Autodesk Inventor part; units mm, degrees
ref_plane "YZ Plane" through (0, 0, 0) normal (1, 0, 0) x (0, 1, 0)
ref_plane "XZ Plane" through (0, 0, 0) normal (0, 1, 0) x (-1, 0, 0)
ref_plane "XY Plane" through (0, 0, 0) normal (0, 0, 1) x (1, 0, 0)
sketch "Sketch1" plane through (0, 0, 0) normal (0, 0, 1) x (1, 0, 0)
  circle A0 centre (0, 0) radius 4
  circle A1 centre (0, 0) radius 40 construction
  circle A2 centre (0, 0) radius 42 construction
  arc A3 (42, 0) -> (-42, 0) centre (0, 0) ccw
  line L0 (-42, 0) -> (-52, 0)
  line L1 (-52, 0) -> (-52, 50)
  line L2 (-52, 50) -> (52, 50)
  line L3 (52, 50) -> (52, 0)
  line L4 (52, 0) -> (42, 0)
  line L5 (-52, 0) -> (-42, 0)
  line L6 (-42, 0) -> (-42, -40)
  line L7 (-42, -40) -> (-52, -40)
  line L8 (-52, -40) -> (-52, 0)
  line L9 (52, 0) -> (42, 0)
  line L10 (42, 0) -> (42, -40)
  line L11 (42, -40) -> (52, -40)
  line L12 (52, -40) -> (52, 0)
  dimension "d0" = 8
  dimension "d1" = 80
  dimension "d2" = 2
  dimension "d3" = 50
  dimension "d4" = 10
  dimension "d5" = 40
extrude "Extrusion1" add sketch "Sketch1" along normal mid plane 7 contours A3 L0 L1 L2 L3 L4 | L4 L12 L11 L10 | L6 L7 L8 L0
sketch "Sketch2" plane through (0, 0, 3.5) normal (0, 0, 1) x (1, 0, 0)
  line L0 (42, 0) -> (42, -40)
  line L1 (42, -40) -> (52, -40)
  line L2 (52, -40) -> (52, 50)
  line L3 (52, 50) -> (-52, 50)
  line L4 (-52, 50) -> (-52, -40)
  line L5 (-52, -40) -> (-42, -40)
  line L6 (-42, -40) -> (-42, 0)
  arc A0 (42, 0) -> (-42, 0) centre (0, 0) ccw
  arc A1 (38, 0) -> (-38, 0) centre (0, 0) ccw
  line L7 (-38, 0) -> (-38, -40)
  line L8 (-38, -40) -> (-42, -40)
  line L9 (38, 0) -> (38, -40)
  line L10 (42, -40) -> (52, -40)
  line L11 (38, -40) -> (42, -40)
  dimension "d11" = 76
extrude "Extrusion2" add sketch "Sketch2" along normal blind 5
sketch "Sketch3" plane through (0, 0, 8.5) normal (0, 0, 1) x (1, 0, 0)
  line L0 (47, -25) -> (-47, -25) construction
  line L1 (-47, -25) -> (-47, 25) construction
  line L2 (-47, 25) -> (47, 25) construction
  line L3 (47, 25) -> (47, -25) construction
  line L4 (47, -25) -> (-47, 25) construction
  line L5 (-47, -25) -> (47, 25) construction
  arc A0 (42, 0) -> (-42, 0) centre (0, 0) ccw construction
  line L6 (-42, -40) -> (-42, 0) construction
  line L7 (42, 0) -> (42, -40) construction
  circle A1 centre (-47, 25) radius 2
  circle A2 centre (-47, -25) radius 2
  circle A3 centre (47, -25) radius 2
  circle A4 centre (47, 25) radius 2
  dimension "d12" = 4
  dimension "d13" = 5
  dimension "d14" = 50
extrude "Extrusion3" cut sketch "Sketch3" against normal through all
sketch "Sketch4" plane through (0, 0, 8.5) normal (0, 0, 1) x (1, 0, 0)
  circle A0 centre (-30, 42) radius 4
  circle A1 centre (30, 42) radius 4
  point P0 (0, 0)
extrude "Extrusion4" cut sketch "Sketch4" against normal through all
sketch "Sketch5" plane through (42, -40, -3.5) normal (0, -1, 0) x (1, 0, 0)
  line L0 (10, 0) -> (10, 12) construction
  line L1 (-4, 12) -> (10, 12) construction
  line L2 (-4, 7) -> (-4, 12)
  line L3 (-4, 7) -> (0, 7)
  line L4 (0, 0) -> (0, 7)
  line L5 (10, 0) -> (0, 0) construction
  line L6 (0, 0) -> (0, 7) construction
  line L7 (0, 3.5) -> (-3, 3.5) construction
  circle A0 centre (-3, 3.5) radius 3
  line L8 (-4, 12) -> (-8, 12)
  line L9 (-80, 12) -> (-4, 12)
  line L10 (-8, 12) -> (-8, 0)
  line L11 (-8, 0) -> (0, 0)
  point P0 (-42, 3.5)
  dimension "d19" = 6
  dimension "d20" = 4
extrude "Extrusion5" add sketch "Sketch5" against normal blind 10
mirror "Mirror1" about plane through (0, 0, 0) normal (1, 0, 0) of "Extrusion5"
fillet "Fillet1" radius 20 2 edges at (52, 50, 2.5) (-52, 50, 2.5)
fillet "Fillet2" radius 5 2 edges at (52, -40, 2.5) (-52, -40, 2.5)
properties part number "frame top"
CAD build for the part. Positions are in the model's coordinates, mm. A direction names the side the tool comes from. Round coordinates to 2 decimals unless told otherwise and drop trailing zeros. Write each loop counter-clockwise with the first axis right and the second up, starting at its lowest first coordinate (ties: lowest second). Pieces come first, ordered by that corner, then holes. Notation, with made-up numbers: (43, 51) -> (49, 51) arc R23 ccw to (49, 65) -> close; hole circle Ø11 at (-9.75, 21). An arc over 180 degrees is marked (long way). Answer in a Markdown table with one row per item. Add a question column.
Item 1: Saw through at C-C, the plane z = 5. Write the cut outline in (x, y).
Item 2: Drop flat-ended pins along their axis: pin 1 Ø9 at (x, y) = (-30, 42) entering from +Z; pin 2 Ø5.5 at (x, z) = (-39, 0) entering from +Y; pin 3 Ø3 at (x, z) = (-5, 0.5) entering from -Y; pin 4 Ø1.5 at (x, z) = (33, 5) entering from +Y. Give the stop position or say it passes through.
Item 3: Saw through at B-B, the plane y = -25. Write the cut outline in (x, z), then the cut area to 3 significant figures.
Item 4: Mould opens along X. For faces 5 (the face through (40, -40, 4)), 6 (the face through (52, -2, 2)), 7 (the face through (-0.92, 41.99, -0.05)) say: pulls with the +X half, pulls with the -X half, needs draft (parallel to the pull), parting line crosses it, or undercut.
Item 5: Saw through at A-A, the plane y = -5. Write the cut outline in (x, z).
Item 6: Drill centre lines: line 1 (Y direction, x = -47, z = 4.5); line 2 (X direction, y = -13.5, z = -2); line 3 (Z direction, x = -16, y = 36.5). Where is each one in solid material? Low to high. Write a range as from..to.
Item 7: Which spindle directions (+Z, -Z, +X, -X, +Y, -Y) get a long thin tool onto all of the face, cutting with end or side? Do faces 1 (the face through (-36, -35, 0)), 2 (the face through (34, -35, 3)), 3 (the face through (38, -15, 6)), 4 (the face through (-42, -15, 0)). Say none if no direction does.
Item 8: Saw through at D-D, the plane y = 40. Write the cut outline in (x, z).
Findings below:
| question | item | result |
|---|---|---|
| 1 | outline | (-52, -35) arc R5 ccw to (-47, -40) -> (-34, -40) -> (-34, -30) -> (-38, -30) -> (-38, 0) arc R38 cw to (38, 0) -> (38, -30) -> (34, -30) -> (34, -40) -> (47, -40) arc R5 ccw to (52, -35) -> (52, 30) arc R20 ccw to (32, 50) -> (-32, 50) arc R20 ccw to (-52, 30) -> close; hole circle Ø4 at (-47, -25); hole circle Ø4 at (-47, 25); hole circle Ø8 at (-30, 42); hole circle Ø8 at (30, 42); hole circle Ø4 at (47, -25); hole circle Ø4 at (47, 25) |
| 2 | pin 1 | stops at z = 8.5 |
| 2 | pin 2 | stops at y = 49.54 |
| 2 | pin 3 | stops at y = 41.49 |
| 2 | pin 4 | stops at y = 50 |
| 3 | outline | (-52, -3.5) -> (-49, -3.5) -> (-49, 8.5) -> (-52, 8.5) -> close; (-45, -3.5) -> (-42, -3.5) -> (-42, 3.5) -> (-38, 3.5) -> (-38, 8.5) -> (-45, 8.5) -> close; (38, 3.5) -> (42, 3.5) -> (42, -3.5) -> (45, -3.5) -> (45, 8.5) -> (38, 8.5) -> close; (49, -3.5) -> (52, -3.5) -> (52, 8.5) -> (49, 8.5) -> close |
| 3 | area | 184 mm^2 |
| 4 | face 5 | needs draft |
| 4 | face 6 | pulls with the +X half |
| 4 | face 7 | undercut |
| 5 | outline | (-52, -3.5) -> (-42, -3.5) -> (-42, 3.5) -> (-38, 3.5) -> (-38, 8.5) -> (-52, 8.5) -> close; (38, 3.5) -> (42, 3.5) -> (42, -3.5) -> (52, -3.5) -> (52, 8.5) -> (38, 8.5) -> close |
| 6 | line 1 | y = -40..-27, -23..23, 27..43.23 |
| 6 | line 2 | x = -52..-42, 42..52 |
| 6 | line 3 | z = 3.5..8.5 |
| 7 | face 1 | -Y |
| 7 | face 2 | +Z, -Z, -Y |
| 7 | face 3 | +Z, -Z |
| 7 | face 4 | -Z |
| 8 | outline | (-49.32, -3.5) -> (-33.46, -3.5) -> (-33.46, 8.5) -> (-49.32, 8.5) -> close; (-26.54, -3.5) -> (-12.81, -3.5) -> (-12.81, 3.5) -> (12.81, 3.5) -> (12.81, -3.5) -> (26.54, -3.5) -> (26.54, 8.5) -> (-26.54, 8.5) -> close; (33.46, -3.5) -> (49.32, -3.5) -> (49.32, 8.5) -> (33.46, 8.5) -> close |
